Geometry: final body of the model. Coordinates: model frame, mm. A direction names the side the tool comes from. Give positions to 0.01 mm unless a question says otherwise; leave off trailing zeros. Write each loop counter-clockwise with the first axis right and the second up, starting at its lowest first coordinate (ties: lowest second). Pieces come first, ordered by that corner, then holes. Notation, with made-up numbers: (-10.5, -38.75) - (34.5, -38.75) arc R8 cw to (34.5, -33.75) - close; hole circle Ø9 at (66, 9). An arc over 180 degrees is marked (long way). Return JSON: item names as keys, results as strings.
from build123d import *

# Parameters (mm, degrees)
SKETCH_1_R      = 2
SKETCH_1_R_2    = 5.03
SKETCH_1_R_3    = 0.8
SKETCH_1_R_4    = 4.03
EXTRUDE_1_DEPTH = 4


with BuildPart() as part:
    # 草图1 → 凸台-拉伸1 (new body)
    with BuildSketch(Plane.XY):
        with BuildLine():
            Line((2.282857143, -22.113571429), (-1.717142857, -22.113571429))
            Line((-1.717142857, -22.113571429), (-1.717142857, -31.613571429))
            Line((-1.717142857, -31.613571429), (-5.717142857, -31.613571429))
            Line((-5.717142857, -31.613571429), (-5.717142857, -39.613571429))
            Line((-5.717142857, -39.613571429), (-1.717142857, -39.613571429))
            Line((-1.717142857, -39.613571429), (13.282857143, -39.613571429))
            Line((13.282857143, -39.613571429), (114.795824144, 18.994967396))
            Line((114.795824144, 18.994967396), (159.545326709, 7.886428571))
            ThreePointArc((159.545326709, 7.886428571), (191.541358842, 15.698516375), (172.851399638, 42.817886077))
            Line((172.851399638, 42.817886077), (136.282857143, 79.386428571))
            ThreePointArc((136.282857143, 79.386428571), (116.282857143, 99.386428571), (96.282857143, 79.386428571))
            Line((96.282857143, 79.386428571), (13.282857143, 49.538084372))
            Line((13.282857143, 49.538084372), (-1.717142857, 49.538084372))
            Line((-1.717142857, 49.538084372), (-1.717142857, 40.886428571))
            Line((-1.717142857, 40.886428571), (2.282857143, 40.886428571))
            Line((2.282857143, 40.886428571), (2.282857143, 42.236428571))
            Line((2.282857143, 42.236428571), (4.882857143, 42.236428571))
            Line((4.882857143, 42.236428571), (4.882857143, 40.886428571))
            Line((4.882857143, 40.886428571), (6.882857143, 40.886428571))
            Line((6.882857143, 40.886428571), (6.882857143, 37.886428571))
            Line((6.882857143, 37.886428571), (4.882857143, 37.886428571))
            Line((4.882857143, 37.886428571), (4.882857143, 36.536428571))
            Line((4.882857143, 36.536428571), (2.282857143, 36.536428571))
            Line((2.282857143, 36.536428571), (2.282857143, 37.886428571))
            Line((2.282857143, 37.886428571), (-1.717142857, 37.886428571))
            Line((-1.717142857, 37.886428571), (-1.717142857, 28.386428571))
            Line((-1.717142857, 28.386428571), (-5.717142857, 28.386428571))
            Line((-5.717142857, 28.386428571), (-5.717142857, 20.386428571))
            Line((-5.717142857, 20.386428571), (-1.717142857, 20.386428571))
            Line((-1.717142857, 20.386428571), (-1.717142857, 10.886428571))
            Line((-1.717142857, 10.886428571), (2.282857143, 10.886428571))
            Line((2.282857143, 10.886428571), (2.282857143, 12.236428571))
            Line((2.282857143, 12.236428571), (4.882857143, 12.236428571))
            Line((4.882857143, 12.236428571), (4.882857143, 10.886428571))
            Line((4.882857143, 10.886428571), (6.882857143, 10.886428571))
            Line((6.882857143, 10.886428571), (6.882857143, 7.886428571))
            Line((6.882857143, 7.886428571), (4.882857143, 7.886428571))
            Line((4.882857143, 7.886428571), (4.882857143, 6.536428571))
            Line((4.882857143, 6.536428571), (2.282857143, 6.536428571))
            Line((2.282857143, 6.536428571), (2.282857143, 7.886428571))
            Line((2.282857143, 7.886428571), (-1.717142857, 7.886428571))
            Line((-1.717142857, 7.886428571), (-1.717142857, -1.613571429))
            Line((-1.717142857, -1.613571429), (-5.717142857, -1.613571429))
            Line((-5.717142857, -1.613571429), (-5.717142857, -9.613571429))
            Line((-5.717142857, -9.613571429), (-1.717142857, -9.613571429))
            Line((-1.717142857, -9.613571429), (-1.717142857, -19.113571429))
            Line((-1.717142857, -19.113571429), (2.282857143, -19.113571429))
            Line((2.282857143, -19.113571429), (2.282857143, -17.763571429))
            Line((2.282857143, -17.763571429), (4.882857143, -17.763571429))
            Line((4.882857143, -17.763571429), (4.882857143, -19.113571429))
            Line((4.882857143, -19.113571429), (6.882857143, -19.113571429))
            Line((6.882857143, -19.113571429), (6.882857143, -22.113571429))
            Line((6.882857143, -22.113571429), (4.882857143, -22.113571429))
            Line((4.882857143, -22.113571429), (4.882857143, -23.463571429))
            Line((4.882857143, -23.463571429), (2.282857143, -23.463571429))
            Line((2.282857143, -23.463571429), (2.282857143, -22.113571429))
        make_face()
        with Locations((32.050124236, 25.489798741)):
            Circle(SKETCH_1_R, mode=Mode.SUBTRACT)
        with Locations((172.851399638, 22.817886077)):
            Circle(SKETCH_1_R_2, mode=Mode.SUBTRACT)
        with Locations((74.16649069, 52.438113656)):
            Circle(SKETCH_1_R, mode=Mode.SUBTRACT)
        with Locations((116.282857143, 73.386428571)):
            Circle(SKETCH_1_R_3, mode=Mode.SUBTRACT)
        with Locations((110.282857143, 79.386428571)):
            Circle(SKETCH_1_R_3, mode=Mode.SUBTRACT)
        with Locations((116.282857143, 79.386428571)):
            Circle(SKETCH_1_R_4, mode=Mode.SUBTRACT)
        with Locations((122.282857143, 79.386428571)):
            Circle(SKETCH_1_R_3, mode=Mode.SUBTRACT)
        with Locations((116.282857143, 85.386428571)):
            Circle(SKETCH_1_R_3, mode=Mode.SUBTRACT)
    extrude(amount=EXTRUDE_1_DEPTH)


solid = part.part
Q1. Set-up query: faces 1 (the flat face through (-1.717, 33, 2)), 2 (the flat face through (-4, -31.614, 2)), 3 (the cylindrical face through (177.5, 20.9, 2)). Return all of +Z, -Z, +X, -X, +Y, -Y with unobstructed straight access to the full face (end or side cutting, diameter ignored); none if empty.
Answer key:
{"face 1": "+Z, -Z, -X, +Y", "face 2": "+Z, -Z, -X", "face 3": "+Z, -Z"}
Q2. Section query A-A, the plane z = 0.7. Count the separate pieces of the cut face and the enclosed holes in it, plus the area to 3 significant figures.
Answer key:
{"separate pieces": "1", "enclosed holes": "8", "area": "13,600 mm^2"}
Q3. Mould query, pull axis X, two halves, no side actions, for faces 4 (the flat face through (-5.717, -6, 2)), 5 (the flat face through (136.857, 13.518, 1.972)), 6 (the flat face through (0, -19.114, 2)). Classes: pulls with the +X half, pulls with the -X half, needs draft (parallel to the pull), parting line crosses it, or undercut.
Answer key:
{"face 4": "pulls with the -X half", "face 5": "undercut", "face 6": "needs draft"}
Q4. Pin query (flat end, axial travel): P1, Ø1.5, axis at y = 11.5, z = 2, coming from the +X side; P2, Ø1, axis at x = 6.5, z = 2.5, coming from the +Y side; P3, Ø1.5, axis at y = 37, z = 3, coming from the +X side. Return the tip coordinate at first contact, or that it passes through.
Answer key:
{"P1": "stops at x = 189.83", "P2": "stops at y = 49.54", "P3": "stops at x = 187.67"}
Q5. Material intervals for probe 1 along Y at (x, z) = (175, 0.35); probe 2 along Y at (x, z) = (123, 0.85); probe 3 along Y at (x, z) = (12, 2.6), sorted ascending. Write a range as [from, to].
Answer key:
{"probe 1": "y = [2.93, 18.27], [27.37, 42.7]", "probe 2": "y = [16.96, 79.03], [79.74, 98.22]", "probe 3": "y = [-39.61, 49.54]"}
Q6. Section query C-C, the plane x = 86. Return the cut outline in (y, z).
Answer key:
{"outline": "(2.37, 0) - (75.69, 0) - (75.69, 4) - (2.37, 4) - close"}
Q7. Section query B-B, the plane x = 38. Return the cut outline in (y, z), plus the area to 3 significant figures.
Answer key:
{"outline": "(-25.34, 0) - (58.43, 0) - (58.43, 4) - (-25.34, 4) - close", "area": "335 mm^2"}
